```python
from build123d import *

# Parameters (mm, degrees)
SKETCH1_R           = 10
SKETCH1_R_2         = 1.5000000000000004
SKETCH1_R_3         = 2.5
BOSS_EXTRUDE1_DEPTH = 2
CUT_EXTRUDE1_START  = -10
SKETCH2_R           = 10
CUT_EXTRUDE1_DEPTH  = 10
BOSS_EXTRUDE3_START = 2
SKETCH4_R           = 4.1899999999999995
SKETCH4_R_2         = 3.667149527921724
BOSS_EXTRUDE3_DEPTH = 2


with BuildPart() as part:
    # Sketch1 → Boss-Extrude1 (new body)
    with BuildSketch(Plane.XY):
        Circle(SKETCH1_R)
        with Locations((0, 7)):
            Circle(SKETCH1_R_2, mode=Mode.SUBTRACT)
        Circle(SKETCH1_R_3, mode=Mode.SUBTRACT)
    extrude(amount=BOSS_EXTRUDE1_DEPTH)

    # Sketch2 → Cut-Extrude1 (cut)
    with BuildSketch(Plane.XY.offset(2).offset(CUT_EXTRUDE1_START)):
        Circle(SKETCH2_R)
        with BuildLine():
            Line((-1.975, 7), (-1.9749999999999994, 3.6953315142216945))
            ThreePointArc((-1.9749999999999994, 3.6953315142216945), (-3.593838477171726, 2.1541645712433404), (-4.1899999999999995, 0))
            ThreePointArc((-4.1899999999999995, 0), (-7.7e-16, -4.1899999999999995), (4.189999999999998, 3.47e-15))
            ThreePointArc((4.189999999999998, 3.47e-15), (3.5938384771717247, 2.1541645712433426), (1.9749999999999959, 3.6953315142216963))
            Line((1.9749999999999959, 3.6953315142216963), (1.974999999999994, 7.000000000000001))
            ThreePointArc((1.974999999999994, 7.000000000000001), (-3.2e-16, 8.974999999999994), (-1.975, 7))
        make_face(mode=Mode.SUBTRACT)
    extrude(amount=CUT_EXTRUDE1_DEPTH, mode=Mode.SUBTRACT)

    # Sketch4 → Boss-Extrude3 (add)
    with BuildSketch(Plane(origin=(0, 0, 0), x_dir=(-1, 0, 0), z_dir=(0, 0, -1)).offset(BOSS_EXTRUDE3_START)):
        with Locations(Location((0, 0, 0), (0, 0, 118.122638153))):
            Circle(SKETCH4_R)
        Circle(SKETCH4_R_2, mode=Mode.SUBTRACT)
    extrude(amount=-BOSS_EXTRUDE3_DEPTH)


solid = part.part
```
Could you check a few things on this model? Use its own coordinates, in mm. A direction names the side the tool comes from. Round coordinates to 2 decimals unless told otherwise and drop trailing zeros. Order: outer loops, then holes, each group sorted by start corner. A loop starts at its lowest first (then second) coordinate and runs counter-clockwise, first axis right, second up. Notation, with made-up numbers: M 10.5,-29.75 L 61.5,-29.75 A32 ccw 61.5,-1.75 Z; hole C 86,56.25 d5. An arc over 180 degrees is marked long. One line per question, with ' | ' between items. Start each with the question number.
(1) Suppose I cut it at D-D on x = 1.75. List the corners of the cut face in (y, z) for me, then the cut area to 3 significant figures.
(2) Please list where these lines run through material, in increasing order: line 1 along Y through (x, z) = (0, 0.9) (3 decimals); line 2 along Y through (x, z) = (0, -1.5); line 3 along Y through (x, z) = (-0.75, 1.5).
(3) Suppose I cut it at B-B on x = 0. List the corners of the cut face in (y, z) for me (3 decimals), then the cut area to 3 significant figures.
(4) For P1, Ø1.5, axis at x = -0.5, y = -0.5, coming from the +Z side; P2, Ø2, axis at y = 4.5, z = 0.5, coming from the -X side; P3, Ø3, axis at x = -0.5, y = 6, coming from the -Z side; P4, Ø1.6, axis at y = 5, z = 1.5, coming from the +X side (3 decimals), each with a flat end and sliding along its axis, tell me the tip position at first contact or that it passes through.
(5) Suppose I cut it at C-C on z = 0.4. List the corners of the cut face in (x, y) for me (3 decimals), then the cut area to 3 significant figures.
(6) Suppose I cut it at A-A on y = 0. List the corners of the cut face in (x, z) for me, then the cut area to 3 significant figures.
(7) For faces 5 (the face through (1.975, 5, 1)), 6 (the face through (-1.975, 5, 1)), 7 (the face through (2, -2, 0)), which set-ups out of +Z, -Z, +X, -X, +Y, -Y let a thin tool reach every point of the face, with its end or its side?
(8) Thinking about a two-plate mould opening in X: for faces 1 (the face through (0.9, 2.5, 2)), 2 (the face through (-3.5, 1.1, -1)), 3 (the face through (0.043, 8.975, 0.986)), 4 (the face through (-0.54, -2.44, 0.99)), which applies, +X half, -X half, draft (parallel to the pull), parting line (faces both ways), or undercut?
Geometry results:
1) outline: M -3.81,-2 L -3.22,-2 L -3.22,0 L -1.79,0 L -1.79,2 L -3.81,2 Z; M 1.79,0 L 3.22,0 L 3.22,-2 L 3.81,-2 L 3.81,0 L 7.92,0 L 7.92,2 L 1.79,2 Z | area: 18.6 mm²
2) line 1: -4.19 to -2.5, 2.5 to 5.5, 8.5 to 8.975 | line 2: -4.19 to -3.67, 3.67 to 4.19 | line 3: -4.12 to -2.38, 2.38 to 5.7, 8.3 to 8.83
3) outline: M -4.19,-2 L -3.667,-2 L -3.667,0 L -2.5,0 L -2.5,2 L -4.19,2 Z; M 2.5,0 L 3.667,0 L 3.667,-2 L 4.19,-2 L 4.19,0 L 5.5,0 L 5.5,2 L 2.5,2 Z; M 8.5,0 L 8.975,0 L 8.975,2 L 8.5,2 Z | area: 12.4 mm²
4) P1: through | P2: x = -2.3 | P3: z = 0 | P4: x = 1.975
5) outline: M -1.975,3.695 A4.19 ccw long 1.975,3.695 L 1.975,7 A1.975 ccw -1.975,7 Z; hole C 0,0 d5; hole C 0,7 d3 | area: 46.3 mm²
6) outline: M -4.19,-2 L -3.67,-2 L -3.67,0 L -2.5,0 L -2.5,2 L -4.19,2 Z; M 2.5,0 L 3.67,0 L 3.67,-2 L 4.19,-2 L 4.19,2 L 2.5,2 Z | area: 8.85 mm²
7) face 5: +Z, -Z, +X, +Y | face 6: +Z, -Z, -X, +Y | face 7: -Z
8) face 1: draft | face 2: undercut | face 3: parting line | face 4: undercut
